Here's the drawing with two shaded views (mm, measured from the low corner). I have some questions. Coordinates: 2 decimals unless noted, no trailing zeros. Write each loop counter-clockwise with the first axis right and the second up, starting at its lowest first coordinate (ties: lowest second). Pieces come first, ordered by that corner, then holes.
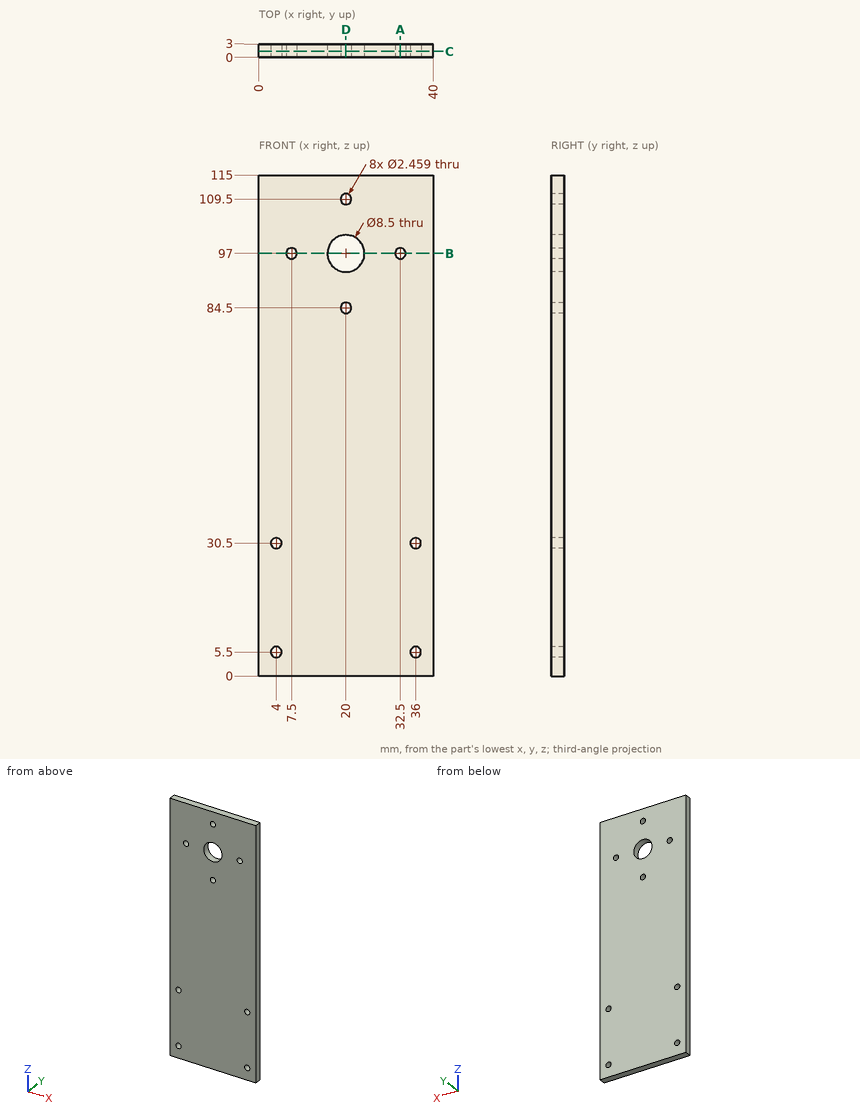
1. Please list where these lines run through material, in increasing order: line 1 along Z through (x, y) = (20, 0.8); line 2 along X through (y, z) = (1.75, 5.5); line 3 along Z through (x, y) = (5, 1.65).
Verdict:
line 1: z = 0 to 83.27, 85.73 to 92.75, 101.25 to 108.27, 110.73 to 115
line 2: x = 0 to 2.77, 5.23 to 34.77, 37.23 to 40
line 3: z = 0 to 4.78, 6.22 to 29.78, 31.22 to 115
2. I want a section at D-D on x = 20. Please give me the cut outline in (y, z).
Verdict:
outline: (0, 0) - (3, 0) - (3, 83.27) - (0, 83.27) - close; (0, 85.73) - (3, 85.73) - (3, 92.75) - (0, 92.75) - close; (0, 101.25) - (3, 101.25) - (3, 108.27) - (0, 108.27) - close; (0, 110.73) - (3, 110.73) - (3, 115) - (0, 115) - close
3. I want a section at B-B on z = 97. Please give me the cut outline in (x, y), plus the area to 3 significant figures.
Verdict:
outline: (0, 0) - (6.27, 0) - (6.27, 3) - (0, 3) - close; (8.73, 0) - (15.75, 0) - (15.75, 3) - (8.73, 3) - close; (24.25, 0) - (31.27, 0) - (31.27, 3) - (24.25, 3) - close; (33.73, 0) - (40, 0) - (40, 3) - (33.73, 3) - close
area: 79.7 mm2
4. I want a section at A-A on x = 32.5. Please give me the cut outline in (y, z).
Verdict:
outline: (0, 0) - (3, 0) - (3, 95.77) - (0, 95.77) - close; (0, 98.23) - (3, 98.23) - (3, 115) - (0, 115) - close
5. I want a section at C-C on y = 1.3. Give the number of separate pieces and of enclosed holes in the cut face, plus the area to 3 significant figures.
Verdict:
separate pieces: 1
enclosed holes: 9
area: 4,510 mm2
